The listing builds one solid part. Answer for the finished solid, in the listing's coordinates (mm). A direction names the side the tool comes from. Give positions to 0.01 mm unless a question says otherwise; leave off trailing zeros. Write each loop counter-clockwise with the first axis right and the second up, starting at its lowest first coordinate (ties: lowest second). Pieces come first, ordered by that corner, then holes. Notation, with made-up numbers: (-24, -15.75) - (22, -15.75) arc R14 ccw to (22, -5.75) - close; hole circle Ø4 at (-33.5, 37). An arc over 180 degrees is marked (long way). Use a Markdown table: item, result. Add a question column.
Autodesk Inventor part; units mm, degrees
ref_plane "YZ Plane" through (0, 0, 0) normal (1, 0, 0) x (0, 1, 0)
ref_plane "XZ Plane" through (0, 0, 0) normal (0, 1, 0) x (-1, 0, 0)
ref_plane "XY Plane" through (0, 0, 0) normal (0, 0, 1) x (1, 0, 0)
sketch "Sketch1" plane through (0, 0, 0) normal (0, 1, 0) x (-1, 0, 0)
  line L0 (100, -50) -> (-100, -50)
  line L1 (-100, -50) -> (-100, 50)
  line L2 (-100, 50) -> (100, 50)
  line L3 (100, 50) -> (100, -50)
  line L4 (100, -50) -> (-100, 50) construction
  line L5 (-100, -50) -> (100, 50) construction
  line L6 (-40, -30) -> (-80, -30)
  line L7 (-50, -50) -> (-70, -50)
  line L8 (-40, -30) -> (-50, -50)
  line L9 (-80, -30) -> (-70, -50)
  line L10 (80, -30) -> (40, -30)
  line L11 (70, -50) -> (50, -50)
  line L12 (80, -30) -> (70, -50)
  line L13 (40, -30) -> (50, -50)
  line L14 (-100, -10) -> (-100, 10)
  line L15 (-80, -20) -> (-80, 20)
  line L16 (-80, -20) -> (-100, -10)
  line L17 (-80, 20) -> (-100, 10)
  line L18 (100, -50) -> (-100, -50)
  line L19 (-100, -50) -> (-130, -50)
  line L20 (-130, -50) -> (-130, 50)
  line L21 (-130, 50) -> (-100, 50)
  line L22 (-100, 50) -> (-100, -50)
  line L23 (-120, -20) -> (-120, 20)
  line L24 (-120, -20) -> (-100, -10)
  line L25 (-120, 20) -> (-100, 10)
  line L26 (-100, 150) -> (-100, 50)
  line L27 (-100, 150) -> (-130, 150)
  line L28 (-130, 150) -> (-130, 50)
  line L29 (-120, 120) -> (-100, 110)
  line L30 (-120, 120) -> (-120, 80)
  line L31 (-120, 80) -> (-100, 90)
  point P0 (0, 0)
  point P1 (-100, 10)
  point P2 (-100, -10)
  point P3 (-70, -50)
  point P4 (-50, -50)
  point P5 (70, -50)
  point P6 (0, 0)
  point P7 (0, 0)
  point P8 (-100, -50)
  dimension "d72" = 200
  dimension "d73" = 100
  dimension "d78" = 20
  dimension "d79" = 40
  dimension "d80" = 20
  dimension "d81" = 10
  dimension "d82" = 20
  dimension "d83" = 40
  dimension "d84" = 20
  dimension "d85" = 10
  dimension "d86" = 120
  dimension "d87" = 30
  dimension "d88" = 0
  dimension "d89" = 0
  dimension "d90" = 40
  dimension "d91" = 20
  dimension "d92" = 20
  dimension "d93" = 10
  dimension "d94" = 40
  dimension "d95" = 0
  dimension "d122" = 30
extrude "Extrusion26" add sketch "Sketch1" along normal blind 12 contours L1 L25 L23 L24 L19 L20 L21 | L21 L28 L27 L26 L29 L30 L31 | L1 L24 L23 L25 | L31 L30 L29 L26
extrude "Extrusion27" cut sketch "Sketch1" along normal blind 6 contours L1 L24 L23 L25 | L31 L30 L29 L26
fillet "Fillet13" radius 2 4 edges at (120, 3, 120) (120, 3, 80) (120, 3, 20) (120, 3, -20)
fillet "Fillet14" radius 6 2 edges at (130, 12, 50) (130, 0, 50)
properties part number "Test2_3DPrint"
1. Consider L1, parallel to Z at x = 112, y = 4.5; L2, parallel to Z at x = 117.5, y = 1.5; L3, parallel to Y at x = 116.5, z = 106. Determine where each line is inside the solid, lowest interval first. Write a range as [from, to].
2. The part is cut by section A-A (x = 105). Give the vertices of the cut face in (y, z), and give its area (3 significant figures).
3. For a pull along X with two mould halves and no side action, classify faces 1 (the flat face through (112, 0, 51)), 2 (the cylindrical face through (128.196, 10.289, 48.6)), 3 (the flat face through (108.673, 2.958, 114.336)) as released by +X, released by -X, zero draft, split by the parting line, or undercut.
4. The part is cut by section C-C (y = 1.75). Give the vertices of the cut face in (x, z), and give its area (3 significant figures).
5. Given P1, Ø4, axis at y = 3.5, z = 17.5, coming from the +X side; P2, Ø2, axis at y = 3, z = 102, coming from the -X side; P3, Ø16, axis at x = 111, z = -2, coming from the -Y side, each flat-ended and moving along its own axis, determine where each tip first touches the part or whether it passes through.
6. Which of the six approach directions +Z, -Z, +X, -X, +Y, -Y give full straight-line access (tool end or side, diameter ignored) to faces 4 (the flat face through (110, 6, 0)), 5 (the flat face through (100, 6, 49))?
Check values:
| question | item | result |
|---|---|---|
| 1 | L1 | z = [-50, -16], [16, 84], [116, 150] |
| 1 | L2 | z = [-50, -18.7], [18.7, 81.3], [118.7, 150] |
| 1 | L3 | y = [6, 12] |
| 2 | outline | (0, -50) - (12, -50) - (12, 150) - (0, 150) - (0, 112.5) - (6, 112.5) - (6, 87.5) - (0, 87.5) - (0, 12.5) - (6, 12.5) - (6, -12.5) - (0, -12.5) - close |
| 2 | area | 2,100 mm2 |
| 3 | face 1 | zero draft |
| 3 | face 2 | released by +X |
| 3 | face 3 | undercut |
| 4 | outline | (100, -50) - (128.24, -50) - (128.24, 150) - (100, 150) - (100, 110) - (117.11, 118.55) arc R2 cw to (120, 116.76) - (120, 83.24) arc R2 cw to (117.11, 81.45) - (100, 90) - (100, 10) - (117.11, 18.55) arc R2 cw to (120, 16.76) - (120, -16.76) arc R2 cw to (117.11, -18.55) - (100, -10) - close |
| 4 | area | 4,460 mm2 |
| 5 | P1 | stops at x = 129.98 |
| 5 | P2 | stops at x = 120 |
| 5 | P3 | stops at y = 6 |
| 6 | face 4 | -Y |
| 6 | face 5 | +Z, -Z, -X, +Y, -Y |
